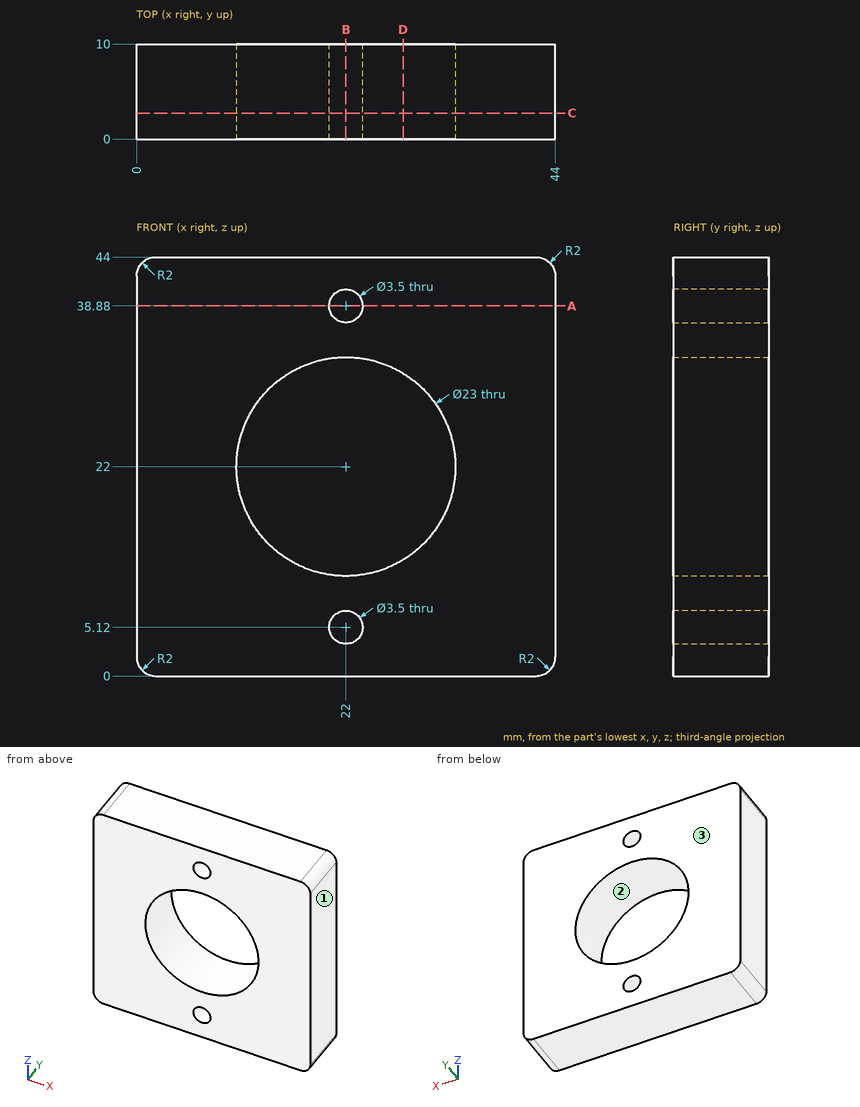
Can you work these out from the drawing? Everything is in mm from the part's minimum corner. Give positions to 0.01 mm unless a question says otherwise; leave off trailing zeros. Loops run counter-clockwise (first coordinate to the right, second up) from the corner with the lowest first, then second, coordinate; pieces in that order, holes last. Notation, with made-up numbers: (66, -16) -> (86, -16) arc R23 cw to (86, 9) -> close; hole circle Ø10 at (89, -40). An arc over 180 degrees is marked (long way). Put each result on its own line as item: value.
(1) Please list where these lines run through material, in increasing order: probe 1 along X at (y, z) = (2, 22); probe 2 along X at (y, z) = (4, 5.12); probe 3 along Z at (x, y) = (21.5, 8.5). Write a range as [from, to].
Computed:
probe 1: [0, 10.5], [33.5, 44]
probe 2: [0, 20.25], [23.75, 44]
probe 3: [0, 3.44], [6.8, 10.51], [33.49, 37.2], [40.56, 44]
(2) Imagine slicing it at B-B on x = 22. Write out the boundary of the cut face in (y, z).
Computed:
outline: (0, 0) -> (10, 0) -> (10, 3.37) -> (0, 3.37) -> close; (0, 6.87) -> (10, 6.87) -> (10, 10.5) -> (0, 10.5) -> close; (0, 33.5) -> (10, 33.5) -> (10, 37.13) -> (0, 37.13) -> close; (0, 40.63) -> (10, 40.63) -> (10, 44) -> (0, 44) -> close
(3) Imagine slicing it at D-D on x = 28. Write out the boundary of the cut face in (y, z).
Computed:
outline: (0, 0) -> (10, 0) -> (10, 12.19) -> (0, 12.19) -> close; (0, 31.81) -> (10, 31.81) -> (10, 44) -> (0, 44) -> close
(4) Imagine slicing it at A-A on z = 38.88. Write out the boundary of the cut face in (x, y), plus the area to 3 significant figures.
Computed:
outline: (0, 0) -> (20.25, 0) -> (20.25, 10) -> (0, 10) -> close; (23.75, 0) -> (44, 0) -> (44, 10) -> (23.75, 10) -> close
area: 405 mm^2
(5) Imagine slicing it at C-C on y = 2.75. Write out the boundary of the cut face in (x, z).
Computed:
outline: (0, 2) arc R2 ccw to (2, 0) -> (42, 0) arc R2 ccw to (44, 2) -> (44, 42) arc R2 ccw to (42, 44) -> (2, 44) arc R2 ccw to (0, 42) -> close; hole circle Ø23 at (22, 22); hole circle Ø3.5 at (22, 5.12); hole circle Ø3.5 at (22, 38.88)
(6) Thinking about a two-plate mould opening in X: for the marked faces 1, 2 and 3, which applies, pulls with the +X half, pulls with the -X half, needs draft (parallel to the pull), parting line crosses it, or undercut?
Computed:
face 1: pulls with the +X half
face 2: undercut
face 3: needs draft
